Read the model definition and answer for the solid it produces. Units are mm, in the model's axes. Coordinates: 2 decimals unless noted, no trailing zeros. Write each loop counter-clockwise with the first axis right and the second up, starting at its lowest first coordinate (ties: lowest second). Pieces come first, ordered by that corner, then holes. Notation, with made-up numbers: (-12, -28) -> (24, -28) arc R19 cw to (24, -18) -> close; hole circle Ø5 at (55.25, 47.5). An arc over 180 degrees is marked (long way). One line per item, written item: value. Start each with the question number.
1. Find section B-B, the plane x = 14. Write down the section's boundary in (y, z).
2. Find section C-C, the plane y = 84. Write down the section's boundary in (x, z).
3. Given P1, Ø1.5, axis at y = 71.5, z = 2.5, coming from the +X side, flat-ended and moving along its own axis, determine where the tip first touches the part or whether it passes through.
4. Consider line 1 along X through (y, z) = (77, 0.75); line 2 along X through (y, z) = (112.5, 2.1); line 3 along Y through (x, z) = (24.5, 2.35). Determine where each line is inside the solid, lowest interval first.
5. Find section A-A, the plane z = 2.4. State how many separate pieces and enclosed holes the cut face has, and give its area (3 significant figures).
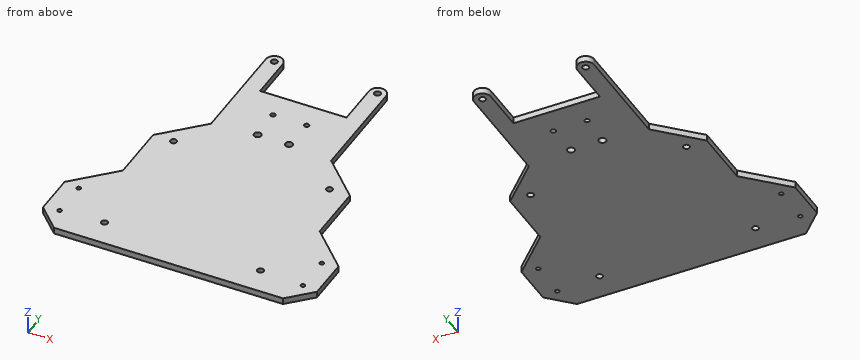
```python
from build123d import *

# Parameters (mm, degrees)
MODEL_R         = 1.75
MODEL_R_2       = 1.15
MODEL_R_3       = 1.5
MODEL_R_4       = 1
EXTRUDE_1_DEPTH = 3


with BuildPart() as part:
    # Model → 凸台-拉伸1 (new body)
    with BuildSketch(Plane.XY):
        with BuildLine():
            Line((-46.68918008, 48.963412214), (-65, 30.652592295))
            Line((-65, 30.652592295), (-65, 10.652592295))
            Line((-65, 10.652592295), (-54.347407705, 0))
            Line((-54.347407705, 0), (54.347407705, 0))
            Line((54.347407705, 0), (65, 10.652592295))
            Line((65, 10.652592295), (65, 30.652592295))
            Line((65, 30.652592295), (46.68918008, 48.963412214))
            Line((46.68918008, 48.963412214), (46.68918008, 76.963412214))
            Line((46.68918008, 76.963412214), (28.5, 95.152592295))
            Line((28.5, 95.152592295), (28.5, 146))
            ThreePointArc((28.5, 146), (24.5, 150), (20.5, 146))
            Line((20.5, 146), (20.5, 125))
            Line((20.5, 125), (-20.5, 125))
            Line((-20.5, 125), (-20.5, 146))
            ThreePointArc((-20.5, 146), (-24.5, 150), (-28.5, 146))
            Line((-28.5, 146), (-28.5, 95.152592295))
            Line((-28.5, 95.152592295), (-46.68918008, 76.963412214))
            Line((-46.68918008, 76.963412214), (-46.68918008, 48.963412214))
        make_face()
        with Locations((7.45, 97.194870059)):
            Circle(MODEL_R, mode=Mode.SUBTRACT)
        with Locations(Location((8, 112.5, 0), (0, 0, 180))):
            Circle(MODEL_R_2, mode=Mode.SUBTRACT)
        with Locations((-24.5, 146)):
            Circle(MODEL_R_3, mode=Mode.SUBTRACT)
        with Locations((37, 13)):
            Circle(MODEL_R_3, mode=Mode.SUBTRACT)
        with Locations((37, 77)):
            Circle(MODEL_R_3, mode=Mode.SUBTRACT)
        with Locations((57.7, 11.852592295)):
            Circle(MODEL_R_4, mode=Mode.SUBTRACT)
        with Locations((-57.7, 11.852592295)):
            Circle(MODEL_R_4, mode=Mode.SUBTRACT)
        with Locations((-57.7, 29.452592295)):
            Circle(MODEL_R_4, mode=Mode.SUBTRACT)
        with Locations((57.7, 29.452592295)):
            Circle(MODEL_R_4, mode=Mode.SUBTRACT)
        with Locations((-37, 77)):
            Circle(MODEL_R_3, mode=Mode.SUBTRACT)
        with Locations((-37, 13)):
            Circle(MODEL_R_3, mode=Mode.SUBTRACT)
        with Locations((24.5, 146)):
            Circle(MODEL_R_3, mode=Mode.SUBTRACT)
        with Locations((-8, 112.5)):
            Circle(MODEL_R_2, mode=Mode.SUBTRACT)
        with Locations((-7.45, 97.194870059)):
            Circle(MODEL_R, mode=Mode.SUBTRACT)
    extrude(amount=EXTRUDE_1_DEPTH)


solid = part.part
```
Answer block:
1. outline: (0, 0) -> (125, 0) -> (125, 3) -> (0, 3) -> close
2. outline: (-39.65, 0) -> (39.65, 0) -> (39.65, 3) -> (-39.65, 3) -> close
3. P1: stops at x = 46.69
4. line 1: x = -46.65 to -38.5, -35.5 to 35.5, 38.5 to 46.65
4. line 2: x = -28.5 to -9.15, -6.85 to 6.85, 9.15 to 28.5
4. line 3: y = 0 to 144.5, 147.5 to 150
5. separate pieces: 1
5. enclosed holes: 14
5. area: 11,900 mm2
